Part print with two shaded views. Sizes in mm from the minimum x, y, z corner. A direction names the side the tool comes from. Give positions to 0.01 mm unless a question says otherwise; leave off trailing zeros. Write each loop counter-clockwise with the first axis right and the second up, starting at its lowest first coordinate (ties: lowest second). Pieces come first, ordered by that corner, then holes. Notation, with made-up numbers: (47.5, 73.5) -> (56.5, 73.5) arc R13 ccw to (56.5, 81.5) -> close; hole circle Ø9 at (31, 54). An arc over 180 degrees is marked (long way). Answer as a JSON object with one key per item and string values.
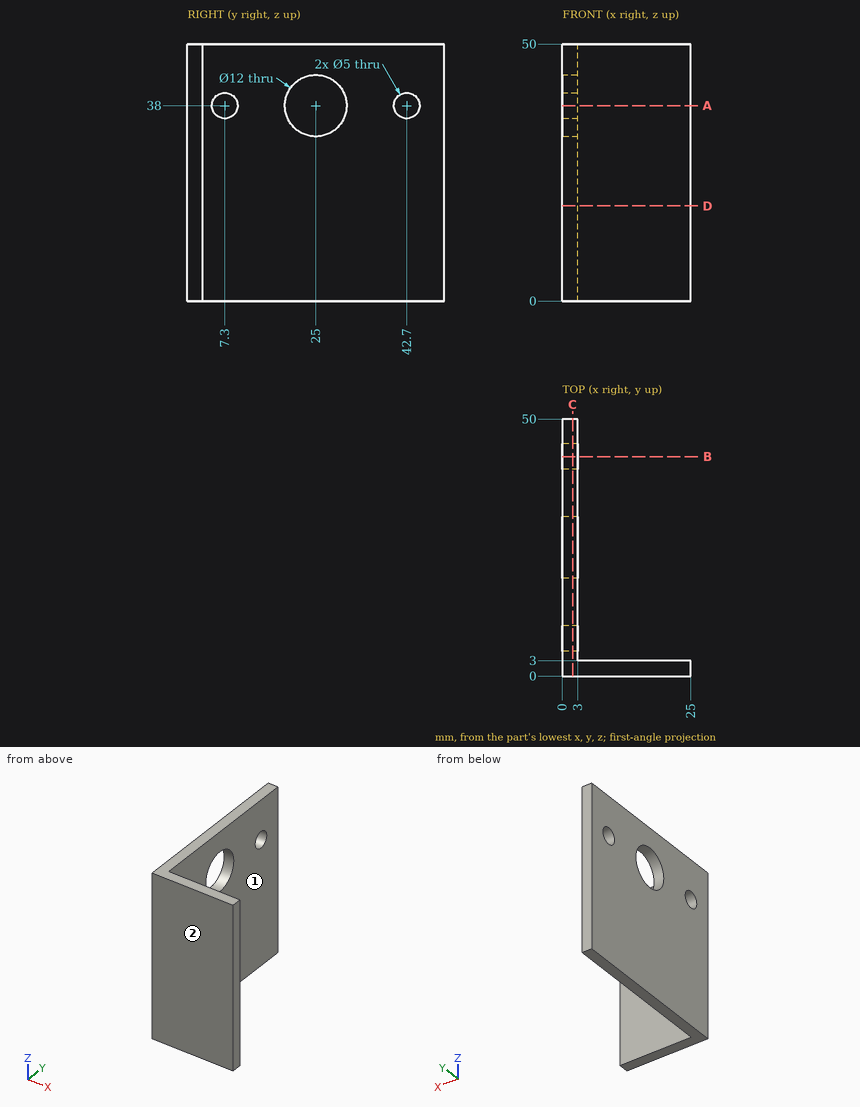
1) Slice it at B-B (y = 42.7). List the corners of the cut face in (x, z), then the cut area to 3 significant figures.
Model answer:
{"outline": "(0, 0) -> (3, 0) -> (3, 35.5) -> (0, 35.5) -> close; (0, 40.5) -> (3, 40.5) -> (3, 50) -> (0, 50) -> close", "area": "135 mm2"}
2) Slice it at D-D (z = 18.5). List the corners of the cut face in (x, y).
Model answer:
{"outline": "(0, 0) -> (25, 0) -> (25, 3) -> (3, 3) -> (3, 50) -> (0, 50) -> close"}
3) Slice it at A-A (z = 38). List the corners of the cut face in (x, y), then the cut area to 3 significant figures.
Model answer:
{"outline": "(0, 0) -> (25, 0) -> (25, 3) -> (3, 3) -> (3, 4.8) -> (0, 4.8) -> close; (0, 9.8) -> (3, 9.8) -> (3, 19) -> (0, 19) -> close; (0, 31) -> (3, 31) -> (3, 40.2) -> (0, 40.2) -> close; (0, 45.2) -> (3, 45.2) -> (3, 50) -> (0, 50) -> close", "area": "150 mm2"}
4) 3-axis set-ups, long thin cutter, end or side, ignore diameter. For the marked faces 1 and 2: which of +Z, -Z, +X, -X, +Y, -Y reach the whole face in a straight line?
Model answer:
{"face 1": "+Z, -Z, +X, +Y", "face 2": "+Z, -Z, +X, -X, -Y"}
5) Pin check, flat tips, straight feed: pin 1 (8 mm diameter, centred on y = 7.3, z = 38, fed in from +X); pin 2 (1 mm diameter, centred on x = 12, z = 42.5, fed in from +Y). Stop position of each tip, or through.
Model answer:
{"pin 1": "stops at x = 3", "pin 2": "stops at y = 3"}
6) Slice it at C-C (x = 2). List the corners of the cut face in (y, z).
Model answer:
{"outline": "(0, 0) -> (50, 0) -> (50, 50) -> (0, 50) -> close; hole circle Ø5 at (7.3, 38); hole circle Ø12 at (25, 38); hole circle Ø5 at (42.7, 38)"}
7) Wall check: probe 1 along Y at (x, z) = (1.2, 38); probe 2 along X at (y, z) = (11.5, 19). Give the ranges that are in metal, low to high.
Model answer:
{"probe 1": "y = 0 to 4.8, 9.8 to 19, 31 to 40.2, 45.2 to 50", "probe 2": "x = 0 to 3"}
